Model file for the job. Use its own axes, mm. A direction names the side the tool comes from. Give positions to 0.01 mm unless a question says otherwise; leave off trailing zeros. Order: outer loops, then holes, each group sorted by start corner. A loop starts at its lowest first (then second) coordinate and runs counter-clockwise, first axis right, second up. Notation, with made-up numbers: (72.5, -19) -> (107.5, -19) arc R19 cw to (107.5, -12) -> close; hole circle Ø8 at (11.25, 56). An arc over 180 degrees is marked (long way). Answer in a Markdown table with one row per item. Add a question column.
from build123d import *

# Parameters (mm, degrees)
F0_R     = 10.9
F1_DEPTH = 5.2
F2_R     = 10


with BuildPart() as f1:
    # F0 (on Top) → F1 (new body)
    with BuildSketch(Plane.XY):
        with BuildLine():
            Line((15.263414, -35.34513), (38.241487, 4.454061))
            ThreePointArc((38.241487, 4.454061), (33.341978, 19.25), (22.978074, 30.891069))
            Line((22.978074, 30.891069), (-22.978074, 30.891069))
            ThreePointArc((-22.978074, 30.891069), (-33.341978, 19.25), (-38.241487, 4.454061))
            Line((-38.241487, 4.454061), (-15.263414, -35.34513))
            ThreePointArc((-15.263414, -35.34513), (0, -38.5), (15.263414, -35.34513))
        make_face()
        Polygon((-5.311622, -15.4), (5.311622, -15.4), (10.623245, -24.6), (5.311622, -33.8), (-5.311622, -33.8), (-10.623245, -24.6), align=None, mode=Mode.SUBTRACT)
        Polygon((-26.615847, 3.1), (-31.92747, 12.3), (-26.615847, 21.5), (-15.992602, 21.5), (-10.68098, 12.3), (-15.992602, 3.1), align=None, mode=Mode.SUBTRACT)
        Circle(F0_R, mode=Mode.SUBTRACT)
        Polygon((15.992602, 21.5), (26.615847, 21.5), (31.92747, 12.3), (26.615847, 3.1), (15.992602, 3.1), (10.68098, 12.3), align=None, mode=Mode.SUBTRACT)
    extrude(amount=F1_DEPTH)

    # F2
    f2_edges = [f1.edges().sort_by_distance(p)[0] for p in [
        (-38.241487, 4.454061, 2.6),
        (-22.978074, 30.891069, 2.6),
        (22.978074, 30.891069, 2.6),
        (38.241487, 4.454061, 2.6),
        (15.263414, -35.34513, 2.6),
        (-15.263414, -35.34513, 2.6),
    ]]
    fillet(f2_edges, radius=F2_R)


solid = f1.part
Item 1: Saw through at A-A on x = 0. List the corners of the cut face in (y, z), plus the area to 3 significant figures.
Item 2: Saw through at B-B on z = 3.5. Give the number of separate pieces and of enclosed holes in the cut face, plus the area to 3 significant figures.
Item 3: Which spindle directions (+Z, -Z, +X, -X, +Y, -Y) get a long thin tool onto all of the face, cutting with end or side? Do faces 1 (the cylindrical face through (33.422, 19.11, 2.564)), 2 (the flat face through (-13.37, 16.96, 2.56)). Say none if no direction does.
Item 4: Pin check, flat tips, straight feed: pin 1 Ø3 at (y, z) = (-26, 2.5) entering from -X; pin 2 Ø2 at (y, z) = (11, 3) entering from +X; pin 3 Ø2.5 at (x, z) = (-21, 3.5) entering from +Y. Stop position of each tip, or through.
Item 5: Saw through at C-C on y = 7. List the corners of the cut face in (x, z), plus the area to 3 significant figures.
Item 6: Saw through at D-D on y = 0. List the corners of the cut face in (x, z).
Item 7: Wall check: line 1 (X direction, y = 14, z = 4.95); line 2 (X direction, y = 4, z = 3.6); line 3 (X direction, y = -21.5, z = 0.35). Give the ranges that are in metal, low to high.
Item 8: Two-plate mould, pull along X, no slides. Class faces 3 (the flat face through (21, 3.1, 3)), 4 (the cylindrical face through (-22.99, 30.22, 2.64)), 5 (the flat face through (8, -11, 5.2)): pulls with the +X half, pulls with the -X half, needs draft (parallel to the pull), parting line crosses it, or undercut.
Evaluation:
| question | item | result |
|---|---|---|
| 1 | outline | (-38.5, 0) -> (-33.8, 0) -> (-33.8, 5.2) -> (-38.5, 5.2) -> close; (-15.4, 0) -> (-10.9, 0) -> (-10.9, 5.2) -> (-15.4, 5.2) -> close; (10.9, 0) -> (30.89, 0) -> (30.89, 5.2) -> (10.9, 5.2) -> close |
| 1 | area | 152 mm2 |
| 2 | separate pieces | 1 |
| 2 | enclosed holes | 4 |
| 2 | area | 2,680 mm2 |
| 3 | face 1 | +Z, -Z, +X, +Y |
| 3 | face 2 | +Z, -Z |
| 4 | pin 1 | stops at x = -21.52 |
| 4 | pin 2 | stops at x = 37.18 |
| 4 | pin 3 | stops at y = 30.88 |
| 5 | outline | (-37.76, 0) -> (-28.87, 0) -> (-28.87, 5.2) -> (-37.76, 5.2) -> close; (-13.74, 0) -> (-8.36, 0) -> (-8.36, 5.2) -> (-13.74, 5.2) -> close; (8.36, 0) -> (13.74, 0) -> (13.74, 5.2) -> (8.36, 5.2) -> close; (28.87, 0) -> (37.76, 0) -> (37.76, 5.2) -> (28.87, 5.2) -> close |
| 5 | area | 149 mm2 |
| 6 | outline | (-35.67, 0) -> (-10.9, 0) -> (-10.9, 5.2) -> (-35.67, 5.2) -> close; (10.9, 0) -> (35.67, 0) -> (35.67, 5.2) -> (10.9, 5.2) -> close |
| 7 | line 1 | x = -35.86 to -30.95, -11.66 to 11.66, 30.95 to 35.86 |
| 7 | line 2 | x = -37.51 to -27.14, -15.47 to -10.14, 10.14 to 15.47, 27.14 to 37.51 |
| 7 | line 3 | x = -23.26 to -8.83, 8.83 to 23.26 |
| 8 | face 3 | undercut |
| 8 | face 4 | pulls with the -X half |
| 8 | face 5 | needs draft |
